Can you work these out from the model? Positions are in its coordinate system, mm. A direction names the side the tool comes from. Give positions to 0.01 mm unless a question says otherwise; leave off trailing zeros. Loops run counter-clockwise (first coordinate to the right, second up) from the corner with the lowest first, then second, coordinate; pieces in that order, holes last. Notation, with made-up numbers: M 52.25,-32 L 89.25,-32 A18 ccw 89.25,-4 Z; hole C 63,-10.75 d9. An arc over 180 degrees is marked long. Put each result on its own line as item: value. Start each with the question number.
1) If we mould it in two halves opening along X, with no side actions, what happens to faces 5 (the cylindrical face through (-13.774, 0.789, -14.309)), 6 (the flat face through (17.5, 0.8, -22.5)), 7 (the flat face through (-12, 3, -3.472))? For each: +X half, -X half, draft (parallel to the pull), parting line (faces both ways), or undercut.
2) Imagine slicing it at D-D (z = 12.5). Write out the boundary of the cut face in (x, y).
3) Imagine slicing it at C-C (x = -11.5). Write out the boundary of the cut face in (y, z), then the cut area to 3 significant figures.
4) Please list where these lines run through material, in increasing order: line 1 along X through (y, z) = (0.6, 15.25); line 2 along Z through (x, y) = (15.5, 0.75); line 3 along Y through (x, z) = (11.5, 12.5). Write a range as from..to.
5) Imagine slicing it at B-B (z = -15.25). Write out the boundary of the cut face in (x, y), then the cut area to 3 significant figures.
6) For faces 1 (the flat face through (-4.185, 3, 2)), 2 (the flat face through (-1, 3, -0.315)), 3 (the flat face through (13.118, 3, 2)), 4 (the flat face through (8, 3, 4.074)), which set-ups out of +Z, -Z, +X, -X, +Y, -Y let a thin tool reach every point of the face, with its end or its side?
7) For P1, Ø0.7, axis at y = 2.5, z = 1.5, coming from the -X side; P2, Ø0.7, axis at x = -2, y = 3, coming from the +Z side; P3, Ø5, axis at x = 7.5, z = 13.5, coming from the +Y side, each with a flat end and sliding along its axis, tell me the tip position at first contact or that it passes through.
8) Imagine slicing it at A-A (y = 2.3). Write out the boundary of the cut face in (x, z), then the cut area to 3 significant figures.
from build123d import *

# Parameters (mm, degrees)
SKETCH1_W        = 36
SKETCH1_H        = 5
SKETCH1_H_2      = 36
SKETCH1_R        = 1.75
PCB_DEPTH        = 1.6
SKETCH2_W        = 5.863870515
SKETCH2_H        = 6.933382723
SKETCH2_W_2      = 7.016073618
SKETCH2_H_2      = 4.389541424
SKETCH2_W_3      = 9.613875512
SKETCH2_H_3      = 4.530712508
COMPONENTS_DEPTH = 2.4
CORNERS_SIZE     = 1


with BuildPart() as part:
    # Sketch1 → PCB (new body)
    # profile 1 of 3: a face of its own
    with BuildSketch(Plane(origin=(0, 0, 0), x_dir=(1, 0, 0), z_dir=(0, 1, 0))):
        with Locations((0, 20.5)):
            Rectangle(SKETCH1_W, SKETCH1_H)
    # profile 2 of 3: a face of its own
    with BuildSketch(Plane(origin=(0, 0, 0), x_dir=(1, 0, 0), z_dir=(0, 1, 0))):
        Rectangle(SKETCH1_W, SKETCH1_H_2)
        with Locations(Location((-15.25, -15.25, 0), (0, 0, 270))):
            Circle(SKETCH1_R, mode=Mode.SUBTRACT)
        with Locations(Location((15.25, -15.25, 0), (0, 0, 270))):
            Circle(SKETCH1_R, mode=Mode.SUBTRACT)
        with Locations(Location((-15.25, 15.25, 0), (0, 0, 270))):
            Circle(SKETCH1_R, mode=Mode.SUBTRACT)
        with Locations(Location((15.25, 15.25, 0), (0, 0, 270))):
            Circle(SKETCH1_R, mode=Mode.SUBTRACT)
    # profile 3 of 3: a face of its own
    with BuildSketch(Plane(origin=(0, 0, 0), x_dir=(1, 0, 0), z_dir=(0, 1, 0))):
        with Locations((0, -20.5)):
            Rectangle(SKETCH1_W, SKETCH1_H)
    extrude(amount=PCB_DEPTH)

    # Sketch2 → Components (add)
    with BuildSketch(Plane(origin=(0, 1.6, 0), x_dir=(1, 0, 0), z_dir=(0, 1, 0))):
        with Locations((-12.422852881, 6.938659117)):
            Rectangle(SKETCH2_W, SKETCH2_H)
        with Locations((-0.676707896, -1.879325534)):
            Rectangle(SKETCH2_W_2, SKETCH2_H_2)
        with Locations((8.311019041, -1.808739992)):
            Rectangle(SKETCH2_W_3, SKETCH2_H_3)
    extrude(amount=COMPONENTS_DEPTH)

    # Corners
    corners_edges = [part.edges().sort_by_distance(p)[0] for p in [
        (-18, 0.8, -23),
        (18, 0.8, -23),
        (18, 0.8, 23),
        (-18, 0.8, 23),
    ]]
    chamfer(corners_edges, length=CORNERS_SIZE)


solid = part.part
Recorded:
1. face 5: undercut
1. face 6: +X half
1. face 7: draft
2. outline: M -18,0 L 18,0 L 18,1.6 L -18,1.6 Z
3. outline: M 0,-23 L 1.6,-23 L 1.6,-10.41 L 4,-10.41 L 4,-3.47 L 1.6,-3.47 L 1.6,23 L 0,23 Z
3. area: 90.2 mm²
4. line 1: -18..-17, -13.5..13.5, 17..18
4. line 2: -23..-16.98, -13.52..13.52, 16.98..23
4. line 3: 0..1.6
5. outline: M -18,0 L -17,0 L -17,1.6 L -18,1.6 Z; M -13.5,0 L 13.5,0 L 13.5,1.6 L -13.5,1.6 Z; M 17,0 L 18,0 L 18,1.6 L 17,1.6 Z
5. area: 46.4 mm²
6. face 1: +Z, -Z, -X, +Y
6. face 2: -Z, -X, +Y
6. face 3: +Z, -Z, +X, +Y
6. face 4: +Z, +X, -X, +Y
7. P1: x = -4.18
7. P2: z = 4.07
7. P3: y = 1.6
8. outline: M -15.35,-10.41 L -9.49,-10.41 L -9.49,-3.47 L -15.35,-3.47 Z; M -4.18,-0.32 L 2.83,-0.32 L 2.83,4.07 L -4.18,4.07 Z; M 3.5,-0.46 L 13.12,-0.46 L 13.12,4.07 L 3.5,4.07 Z
8. area: 115 mm²
